```python
from build123d import *

# Parameters (mm, degrees)
SKETCH1_W           = 47.63
SKETCH1_H           = 51.3
SKETCH1_R           = 2.15
BOSS_EXTRUDE1_DEPTH = 42.6
SKETCH2_R           = 9.525
CUT_EXTRUDE1_DEPTH  = 98.066930034
SKETCH3_W           = 32.23
SKETCH3_H           = 57.048665503
CUT_EXTRUDE2_DEPTH  = 0.38


with BuildPart() as part:
    # Sketch1 → Boss-Extrude1 (new body)
    with BuildSketch(Plane(origin=(0, 0, 0), x_dir=(1, 0, 0), z_dir=(0, 1, 0))):
        with Locations((-46.7225, 12.267391304)):
            Rectangle(SKETCH1_W, SKETCH1_H)
        with Locations(Location((-66.5475, 31.317391304, 0), (0, 0, 270))):
            Circle(SKETCH1_R, mode=Mode.SUBTRACT)
        with Locations(Location((-26.8975, 31.317391304, 0), (0, 0, 270))):
            Circle(SKETCH1_R, mode=Mode.SUBTRACT)
        with Locations(Location((-66.5475, -6.782608696, 0), (0, 0, 270))):
            Circle(SKETCH1_R, mode=Mode.SUBTRACT)
        with Locations(Location((-26.8975, -6.782608696, 0), (0, 0, 270))):
            Circle(SKETCH1_R, mode=Mode.SUBTRACT)
    extrude(amount=BOSS_EXTRUDE1_DEPTH)

    # Sketch2 → Cut-Extrude1 (cut, through all)
    with BuildSketch(Plane.XY.offset(13.382608696)):
        with Locations((-46.7225, 22.23)):
            Circle(SKETCH2_R)
    extrude(amount=-CUT_EXTRUDE1_DEPTH, mode=Mode.SUBTRACT)

    # Sketch3 → Cut-Extrude2 (cut)
    with BuildSketch(Plane.XZ):
        with Locations((-46.7225, -11.363905652)):
            Rectangle(SKETCH3_W, SKETCH3_H)
    extrude(amount=-CUT_EXTRUDE2_DEPTH, mode=Mode.SUBTRACT)


solid = part.part
```
For this review, take the finished solid that the model builds, in its own axes (mm). A direction names the side the tool comes from. Give positions to 0.01 mm unless a question says otherwise; leave off trailing zeros. Order: outer loops, then holes, each group sorted by start corner. A loop starts at its lowest first (then second) coordinate and runs counter-clockwise, first axis right, second up.
1) The part is to be moulded in two halves that separate along Z. For faces 3 (the face through (-64.416, 21.002, 6.503)), 4 (the face through (-47, 12, 13.383)), 5 (the face through (-70.538, 21, -12)), say which applies: released by +Z, released by -Z, zero draft, split by the parting line, or undercut.
2) Take a section at D-D (x = -55). Give the boundary of the cut face in (y, z).
3) Wall thickness on line 1 (X direction, y = 40, z = 7); line 2 (Z direction, x = -25, y = 20.5); line 3 (X direction, y = 31, z = -21): over which ranges is each line inside the solid? List them lowest first.
4) Take a section at C-C (z = 5.5). State how many separate pieces and enclosed holes the cut face has, then the cut area to 3 significant figures.
5) Insertion check: pin 1 (4 mm diameter, centred on x = -50, z = 4.5, fed in from -Y); pin 2 (4 mm diameter, centred on x = -66.55, z = -31.32, fed in from -Y). Each pin has a flat end and moves straight along its axis. Give the tip position at first contact, or say it passes through.
6) For faces 1 (the face through (-47, 0.38, -12)), 2 (the face through (-47, 12, -37.917)), list the 3-axis set-ups (+Z, -Z, +X, -X, +Y, -Y) from which the entire face can be reached by the end or side of a thin tool; tool diameter is ignored.
7) Take a section at B-B (y = 22.23). Give the boundary of the cut face in (x, z), then the cut area to 3 significant figures.
Derived:
1. face 3: undercut
1. face 4: released by +Z
1. face 5: zero draft
2. outline: (0.38, -37.92) - (17.52, -37.92) - (17.52, 13.38) - (0.38, 13.38) - close; (26.94, -37.92) - (42.6, -37.92) - (42.6, 13.38) - (26.94, 13.38) - close
3. line 1: x = -70.54 to -68.69, -64.41 to -29.04, -24.76 to -22.91
3. line 2: z = -37.92 to -32.33, -30.31 to 5.77, 7.79 to 13.38
3. line 3: x = -70.54 to -50.44, -43.01 to -22.91
4. separate pieces: 3
4. enclosed holes: 1
4. area: 1,440 mm2
5. pin 1: stops at y = 0.38
5. pin 2: passes through
6. face 1: +Z, -Z, -Y
6. face 2: -Z, +X, -X, +Y, -Y
7. outline: (-70.54, -37.92) - (-56.25, -37.92) - (-56.25, 13.38) - (-70.54, 13.38) - close; (-37.2, -37.92) - (-22.91, -37.92) - (-22.91, 13.38) - (-37.2, 13.38) - close; hole circle Ø4.3 at (-66.55, -31.32); hole circle Ø4.3 at (-66.55, 6.78); hole circle Ø4.3 at (-26.9, -31.32); hole circle Ø4.3 at (-26.9, 6.78)
7. area: 1,410 mm2
